Autodesk Inventor part; units mm, degrees
ref_plane "YZ Plane" through (0, 0, 0) normal (1, 0, 0) x (0, 1, 0)
ref_plane "XZ Plane" through (0, 0, 0) normal (0, 1, 0) x (-1, 0, 0)
ref_plane "XY Plane" through (0, 0, 0) normal (0, 0, 1) x (1, 0, 0)
ref_plane "Work Plane1" through (82.6105, 192.6947, -14.7678) normal (0, 0, 1) x (1, 0, 0)
sketch "Sketch1" plane through (82.6105, 192.6947, -14.7678) normal (0, 0, 1) x (1, 0, 0)
  line L0 (76.2, 79.375) -> (76.2, 31.115)
  arc A0 (-66.9925, 57.785) -> (-58.7375, 57.785) centre (-62.865, 57.785) ccw
  line L1 (-66.9925, 57.785) -> (-66.9925, 79.375)
  line L2 (-58.7375, 57.785) -> (-58.7375, 79.375)
  line L3 (-76.2, 79.375) -> (-66.9925, 79.375)
  line L4 (0, 79.375) -> (0, 48.4751) construction
  line L5 (58.7375, 57.785) -> (58.7375, 79.375)
  line L6 (66.9925, 57.785) -> (66.9925, 79.375)
  arc A1 (58.7375, 57.785) -> (66.9925, 57.785) centre (62.865, 57.785) ccw
  line L7 (-58.7375, 79.375) -> (58.7375, 79.375)
  line L8 (66.9925, 79.375) -> (76.2, 79.375)
  line L9 (-60.325, 41.275) -> (-60.325, 31.115)
  line L10 (-60.325, 41.275) -> (60.325, 41.275)
  line L11 (60.325, 41.275) -> (60.325, 31.115)
  line L12 (-76.2, 79.375) -> (-76.2, 31.115)
  circle A2 centre (0, 50.275) radius 3.5
  circle A3 centre (5.5, 50.275) radius 1
  circle A4 centre (-5.5, 50.275) radius 1
  line L13 (-60.325, 31.115) -> (-76.2, 31.115)
  line L14 (60.325, 31.115) -> (76.2, 31.115)
  point P0 (-82.6105, -192.6947)
  point P1 (0, 0)
  dimension "d1" = 76.2
  dimension "d4" = 8.255
  dimension "d10" = 152.4
  dimension "d11" = 7
  dimension "d12" = 9
  dimension "d13" = 2
  dimension "d14" = 5.5
  dimension "d15" = 2
  dimension "d16" = 5.5
  dimension "d17" = 57.785
extrude "Extrusion1" add sketch "Sketch1" along normal blind 8.66
chamfer "Chamfer1" distance 1.5875 angle 45 8 edges at (158.8105, 223.8097, -10.4378) (141.348, 272.0697, -10.4378) (158.8105, 272.0697, -10.4378) (6.4105, 223.8097, -10.4378) (6.4105, 272.0697, -10.4378) (15.618, 272.0697, -10.4378) (23.873, 272.0697, -10.4378) (149.603, 272.0697, -10.4378)
properties part number "Lower Bracket"
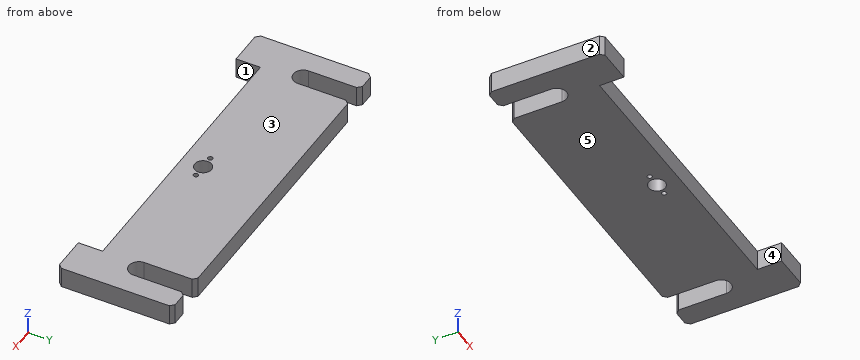
Geometry: final body of the model. Coordinates: model frame, mm. Face numbers are marked on the shaded views. A direction names the side the tool comes from. Coordinates: 2 decimals unless noted, no trailing zeros. Write each loop counter-clockwise with the first axis right and the second up, starting at its lowest first coordinate (ties: lowest second). Pieces come first, ordered by that corner, then holes. Notation, with made-up numbers: M 57.25,-4.5 L 116.25,-4.5 A28 cw 116.25,30.5 Z; hole C 17.25,68.25 d2. An arc over 180 degrees is marked long. Answer as CSV lines item,"result". Start each with the question number.
Q1. Mould query, pull axis X, two halves, no side actions, for the marked faces 1, 2 and 3. Classes: released by +X, released by -X, zero draft, split by the parting line, or undercut.
Q2. Cut plane D-D on x = 129. Return the cut outline in (y, z), then the cut area to 3 significant figures.
Q3. Cut plane C-C on z = -13.25. Return the cut outline in (x, y) (1 decimal), then the cut area to 3 significant figures.
Q4. Reachability of the marked faces 4 and 5 from +Z, -Z, +X, -X, +Y, -Y: full face, straight path, thin tool, end or side. Return the list, or none.
Q5. Pin query (flat end, axial travel): P1, Ø1, axis at x = 49.5, z = -12.5, coming from the -Y side; P2, Ø6.5, axis at x = 82.61, y = 242.97, coming from the -Z side. Return the tip coordinate at first contact, or that it passes through.
Q6. Cut plane A-A on y = 254. Return the cut outline in (x, z).
Q7. Line query: line 1 (X direction, y = 267, z = -13); line 2 (X direction, y = 250, z = -14); line 3 (X direction, y = 233, z = -9.25). Output: solid intervals per line, ascending. Write a range as from..to.
Q8. Cut plane B-B on y = 228. Return the cut outline in (x, z), then the cut area to 3 significant figures.
Findings below:
1,face 1,"undercut"
1,face 2,"released by -X"
1,face 3,"zero draft"
2,outline,"M 233.97,-14.77 L 272.07,-14.77 L 272.07,-6.11 L 233.97,-6.11 Z"
2,area,"330 mm2"
3,outline,"M 6.4,225.4 L 8,223.8 L 22.3,223.8 L 22.3,234 L 142.9,234 L 142.9,223.8 L 157.2,223.8 L 158.8,225.4 L 158.8,270.5 L 157.2,272.1 L 151.2,272.1 L 149.6,270.5 L 149.6,250.5 A4.1 cw 141.3,250.5 L 141.3,270.5 L 139.8,272.1 L 25.5,272.1 L 23.9,270.5 L 23.9,250.5 A4.1 cw 15.6,250.5 L 15.6,270.5 L 14,272.1 L 8,272.1 L 6.4,270.5 Z; hole C 77.1,243 d2; hole C 82.6,243 d7; hole C 88.1,243 d2"
3,area,"5,660 mm2"
4,face 4,"+Z, -Z, -Y"
4,face 5,"-Z, +X, -X, +Y, -Y"
5,P1,"stops at y = 233.97"
5,P2,"passes through"
6,outline,"M 6.41,-14.77 L 15.62,-14.77 L 15.62,-6.11 L 6.41,-6.11 Z; M 23.87,-14.77 L 141.35,-14.77 L 141.35,-6.11 L 23.87,-6.11 Z; M 149.6,-14.77 L 158.81,-14.77 L 158.81,-6.11 L 149.6,-6.11 Z"
7,line 1,"x = 6.41..15.62, 23.87..141.35, 149.6..158.81"
7,line 2,"x = 6.41..15.65, 23.85..141.38, 149.58..158.81"
7,line 3,"x = 6.41..22.29, 142.94..158.81"
8,outline,"M 6.41,-14.77 L 22.29,-14.77 L 22.29,-6.11 L 6.41,-6.11 Z; M 142.94,-14.77 L 158.81,-14.77 L 158.81,-6.11 L 142.94,-6.11 Z"
8,area,"275 mm2"
